Can you work these out from the model? Positions are in its coordinate system, mm. Face numbers are marked on the shaded views. Give positions to 0.01 mm unless a question says otherwise; leave off trailing zeros. Order: outer loops, then holes, each group sorted by start corner. A loop starts at its lowest first (then second) coordinate and runs counter-clockwise, first axis right, second up. Notation, with made-up numbers: (70, 75) - (108, 75) arc R22 ccw to (108, 97) - close; hole circle Ø2 at (-32, 65). An arc over 180 degrees is marked (long way). Answer as a JSON object with one key per item and string values.
```python
from build123d import *

# Parameters (mm, degrees)
SKETCH1_R                = 20
BOSS_EXTRUDE1_DEPTH      = 50
SKETCH2_R                = 40
BOSS_EXTRUDE2_DEPTH      = 5
CHAMFER1_SIZE            = 2
SKETCH3_R                = 2.5
CUT_EXTRUDE1_DEPTH       = 120.268604419
CIRPATTERN1_COUNT        = 6
FILLET1_R                = 3
MIRROR2_COPY_1_SKETCH_R  = 2.5
MIRROR2_COPY_1_DEPTH     = 120.268604419
MIRROR2_COPY_2_SKETCH_R  = 2.5
MIRROR2_COPY_2_DEPTH     = 120.268604419
MIRROR2_COPY_3_SKETCH_R  = 2.5
MIRROR2_COPY_3_DEPTH     = 120.268604419
MIRROR2_COPY_4_SKETCH_R  = 2.5
MIRROR2_COPY_4_DEPTH     = 120.268604419
MIRROR2_COPY_5_SKETCH_R  = 2.5
MIRROR2_COPY_5_DEPTH     = 120.268604419
CHAMFER1_OF_MIRROR2_SIZE = 2
FILLET1_OF_MIRROR2_R     = 3


with BuildPart() as part:
    # Sketch1 → Boss-Extrude1 (new, symmetric)
    with BuildSketch(Plane.XY):
        Circle(SKETCH1_R)
    extrude(amount=BOSS_EXTRUDE1_DEPTH, both=True)

    # Sketch2 → Boss-Extrude2 (add)
    with BuildSketch(Plane.XY.offset(50)):
        Circle(SKETCH2_R)
    boss_extrude2 = extrude(amount=BOSS_EXTRUDE2_DEPTH)

    # Chamfer1
    chamfer1_edges = [part.edges().sort_by_distance(p)[0] for p in [
        (-40, 0, 55),
    ]]
    chamfer(chamfer1_edges, length=CHAMFER1_SIZE)

    # Sketch3 → Cut-Extrude1 (cut, through all)
    with BuildSketch(Plane.XY.offset(55)):
        with Locations((0, 30)):
            Circle(SKETCH3_R)
    cut_extrude1 = extrude(amount=-CUT_EXTRUDE1_DEPTH, mode=Mode.SUBTRACT)

    # CirPattern1: Cut-Extrude1 ×6 about axis
    cirpattern1_axis = Axis((0, 0, 0), (0, 0, 1))
    for i in range(1, CIRPATTERN1_COUNT):
        add(cut_extrude1.rotate(cirpattern1_axis, i * 360 / CIRPATTERN1_COUNT), mode=Mode.SUBTRACT)

    # Fillet1
    fillet1_edges = [part.edges().sort_by_distance(p)[0] for p in [
        (-40, 0, 50),
    ]]
    fillet(fillet1_edges, radius=FILLET1_R - 0.0001)  # a hair under: the kernel refuses the full size

    # Sketch5 → CBORE for M12 Hex Head Bolt1 (revolve, cut)
    with BuildSketch(Plane(origin=(0, 0, 55), x_dir=(0, -1, 0), z_dir=(1, 0, 0))):
        Polygon((0, 0), (0, 110), (6.5, 110), (6.5, 7.95), (11.89, 7.95), (11.89, 0.025), (11.915, 0), align=None)
    cbore_for_m12_hex_head_bolt1 = revolve(axis=Axis((0, 0, 61.35), (0, 0, -1)), mode=Mode.SUBTRACT)

    # Mirror2: Boss-Extrude2, Cut-Extrude1, CBORE for M12 Hex Head Bolt1 across plane
    add(boss_extrude2.mirror(Plane.XY))
    add(cut_extrude1.mirror(Plane.XY), mode=Mode.SUBTRACT)
    add(cbore_for_m12_hex_head_bolt1.mirror(Plane.XY), mode=Mode.SUBTRACT)

    # Mirror2 copy 1 sketch → Mirror2 copy 1 (cut, through all)
    with BuildSketch(Plane(origin=(0, 0, -55), x_dir=(0.5000000000000001, 0.8660254037844386, 0), z_dir=(0, 0, -1))):
        with Locations((0, -30)):
            Circle(MIRROR2_COPY_1_SKETCH_R)
    extrude(amount=-MIRROR2_COPY_1_DEPTH, mode=Mode.SUBTRACT)

    # Mirror2 copy 2 sketch → Mirror2 copy 2 (cut, through all)
    with BuildSketch(Plane(origin=(0, 0, -55), x_dir=(-0.4999999999999998, 0.8660254037844387, 0), z_dir=(0, 0, -1))):
        with Locations((0, -30)):
            Circle(MIRROR2_COPY_2_SKETCH_R)
    extrude(amount=-MIRROR2_COPY_2_DEPTH, mode=Mode.SUBTRACT)

    # Mirror2 copy 3 sketch → Mirror2 copy 3 (cut, through all)
    with BuildSketch(Plane(origin=(0, 0, -55), x_dir=(-1, 0, 0), z_dir=(0, 0, -1))):
        with Locations((0, -30)):
            Circle(MIRROR2_COPY_3_SKETCH_R)
    extrude(amount=-MIRROR2_COPY_3_DEPTH, mode=Mode.SUBTRACT)

    # Mirror2 copy 4 sketch → Mirror2 copy 4 (cut, through all)
    with BuildSketch(Plane(origin=(0, 0, -55), x_dir=(-0.5000000000000004, -0.8660254037844384, 0), z_dir=(0, 0, -1))):
        with Locations((0, -30)):
            Circle(MIRROR2_COPY_4_SKETCH_R)
    extrude(amount=-MIRROR2_COPY_4_DEPTH, mode=Mode.SUBTRACT)

    # Mirror2 copy 5 sketch → Mirror2 copy 5 (cut, through all)
    with BuildSketch(Plane(origin=(0, 0, -55), x_dir=(0.5000000000000001, -0.8660254037844386, 0), z_dir=(0, 0, -1))):
        with Locations((0, -30)):
            Circle(MIRROR2_COPY_5_SKETCH_R)
    extrude(amount=-MIRROR2_COPY_5_DEPTH, mode=Mode.SUBTRACT)

    # Chamfer1 of Mirror2
    chamfer1_of_mirror2_edges = [part.edges().sort_by_distance(p)[0] for p in [
        (-40, 0, -55),
    ]]
    chamfer(chamfer1_of_mirror2_edges, length=CHAMFER1_OF_MIRROR2_SIZE)

    # Fillet1 of Mirror2
    fillet1_of_mirror2_edges = [part.edges().sort_by_distance(p)[0] for p in [
        (-40, 0, -50),
    ]]
    fillet(fillet1_of_mirror2_edges, radius=FILLET1_OF_MIRROR2_R - 0.0001)  # a hair under: the kernel refuses the full size


solid = part.part
```
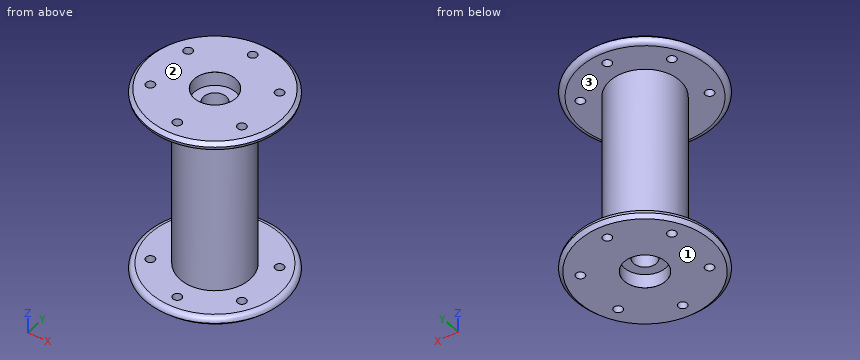
Q1. We'd pull the mould along Z, two halves only. Please class the marked faces 1, 2 and 3: released by +Z, released by -Z, zero draft, split by the parting line, or undercut.
Recorded:
{"face 1": "released by -Z", "face 2": "released by +Z", "face 3": "undercut"}
Q2. If we section it at B-B, the plane z = 19.5: Please give me the cut outline in (x, y).
Recorded:
{"outline": "circle Ø40 at (0, 0); hole circle Ø13 at (0, 0)"}
Q3. I need wall thicknesses on L1, parallel to Y at x = 0, z = 53; L2, parallel to Z at x = 31.5, y = 2; L3, parallel to Z at x = 4.5, y = 7.5. Which ranges of each line are inside material? Lowest first, please.
Recorded:
{"L1": "y = -40 to -32.5, -27.5 to -11.89, 11.89 to 27.5, 32.5 to 40", "L2": "z = -55 to -50, 50 to 55", "L3": "z = -47.05 to 47.05"}
Q4. I'm going to push flat-ended pins straight in: pin 1 Ø10 at (x, z) = (17.5, 39.5) entering from -Y; pin 2 Ø1.5 at (y, z) = (-13, -5) entering from -X; pin 3 Ø4 at (x, z) = (9.5, -21) entering from +Y. Where does each tip first touch, or does it pass through?
Recorded:
{"pin 1": "stops at y = -15.61", "pin 2": "stops at x = -15.81", "pin 3": "stops at y = 18.54"}
Q5. If we section it at A-A, the plane x = 0: Count the separate pieces of the cut face and the enclosed holes in it, then the cut area to 3 significant figures.
Recorded:
{"separate pieces": "6", "enclosed holes": "0", "area": "3,080 mm^2"}
